Input: part model. Units: mm. Frame: model coordinates. A direction names the side the tool comes from. Round coordinates to 2 decimals unless told otherwise and drop trailing zeros. Order: outer loops, then holes, each group sorted by start corner. A loop starts at its lowest first (then second) coordinate and runs counter-clockwise, first axis right, second up. Notation, with made-up numbers: (12.5, 47) -> (69.5, 47) arc R12 ccw to (69.5, 52) -> close; hole circle Ø3 at (-24, -10.5). An arc over 180 degrees is marked (long way). Answer as CSV lines item,"result". Start each with the question number.
1) Section query A-A, the plane y = 40.5. Output: boundary loops of the cut face in (x, z).
2) Section query B-B, the plane z = 22. Output: boundary loops of the cut face in (x, y).
3) Mould query, pull axis Y, two halves, no side actions, for faces 5 (the face through (26, 3, -10)), 6 (the face through (32.266, 1.479, -13.562)), 7 (the face through (-38.22, 30.225, -8.997)). Classes: +Y half, -Y half, draft (parallel to the pull), parting line (faces both ways), or undercut.
4) Access query for faces 1 (the face through (-40.82, 22.72, -14.99)), 2 (the face through (-31, 3, 13)), 3 (the face through (28.564, 26.856, 9.951)), 4 (the face through (-37.038, 26.856, -6.273)). Directions: +Z, -Z, +X, -X, +Y, -Y. A direction counts if a zero-diameter tool reaches every point of the face in a straight line with its end or side. Return the directions, or none.
5) First-contact query: P1, Ø3, axis at y = 17, z = -10.5, coming from the -X side; P2, Ø4, axis at x = 22, y = 10.5, coming from the -Z side; P3, Ø19, axis at x = 29, z = -21, coming from the +Y side. Flat tips, straight axial feed; report the tip coordinate or a pass-through.
6) Line query: L1, parallel to Y at x = 16, z = -20; L2, parallel to Y at x = -28.5, z = 9; L3, parallel to X at y = 7.5, z = -9. Output: solid intervals per line, ascending.
7) Section query C-C, the plane x = -28. Output: boundary loops of the cut face in (y, z).
```python
from build123d import *

# Parameters (mm, degrees)
SKETCH1_R           = 0.5
BOSS_EXTRUDE1_DEPTH = 3
BOSS_EXTRUDE2_START = 30
SKETCH2_W           = 60
SKETCH2_H           = 40
SKETCH2_R           = 1.689490446
SKETCH2_W_2         = 41
SKETCH2_H_2         = 20.5
BOSS_EXTRUDE2_DEPTH = 3
BOSS_EXTRUDE3_START = -23.72
SKETCH2_2_W         = 60
SKETCH2_2_H         = 40
SKETCH2_2_R         = 1.689490446
SKETCH2_2_W_2       = 41
SKETCH2_2_H_2       = 20.5
BOSS_EXTRUDE3_DEPTH = 3
CUT_EXTRUDE1_DEPTH  = 10


with BuildPart() as part:
    # Sketch1 → Boss-Extrude1 (new body)
    with BuildSketch(Plane(origin=(0, 0, 0), x_dir=(1, 0, 0), z_dir=(0, 1, 0))):
        with BuildLine():
            ThreePointArc((7.77744177, 34.124938088), (-19.979563219, 28.73703279), (-34.697157454, 4.594264319))
            Line((-34.697157454, 4.594264319), (-39.463419759, 15.576857865))
            Line((-39.463419759, 15.576857865), (-42.291947314, 14.577141972))
            Line((-42.291947314, 14.577141972), (-34.916382331, -2.417900937))
            ThreePointArc((-34.916382331, -2.417900937), (-32.106828614, -13.933827771), (-25.614551861, -23.85151427))
            Line((-25.614551861, -23.85151427), (-18.322186149, -40.654846416))
            Line((-18.322186149, -40.654846416), (-15.576857865, -39.463419759))
            Line((-15.576857865, -39.463419759), (-20.34312017, -28.480826213))
            ThreePointArc((-20.34312017, -28.480826213), (7.343177958, -34.221013098), (30.237043308, -17.627286007))
            Line((30.237043308, -17.627286007), (30.950523486, -19.271312771))
            Line((30.950523486, -19.271312771), (33.702537367, -18.076984677))
            Line((33.702537367, -18.076984677), (32.005152982, -14.165810341))
            ThreePointArc((32.005152982, -14.165810341), (32.106828614, 13.933827771), (11.51335986, 33.052118612))
            Line((11.51335986, 33.052118612), (9.815975474, 36.963292947))
            Line((9.815975474, 36.963292947), (7.063961593, 35.768964852))
            Line((7.063961593, 35.768964852), (7.77744177, 34.124938088))
        make_face()
        with Locations(Location((0, -16.15, 0), (0, 0, 270))):
            Circle(SKETCH1_R, mode=Mode.SUBTRACT)
        with BuildLine():
            ThreePointArc((0, -12.65), (0.5, -13.15), (0, -13.65))
            ThreePointArc((0, -13.65), (-0.5, -13.15), (0, -12.65))
        make_face(mode=Mode.SUBTRACT)
        with BuildLine():
            ThreePointArc((0, -9.65), (0.5, -10.15), (0, -10.65))
            ThreePointArc((0, -10.65), (-0.5, -10.15), (0, -9.65))
        make_face(mode=Mode.SUBTRACT)
        with BuildLine():
            ThreePointArc((0, -6.005210608), (0.5, -6.505210608), (0, -7.005210608))
            ThreePointArc((0, -7.005210608), (-0.5, -6.505210608), (0, -6.005210608))
        make_face(mode=Mode.SUBTRACT)
        with Locations(Location((-16.15, 0, 0), (0, 0, 270))):
            Circle(SKETCH1_R, mode=Mode.SUBTRACT)
        with BuildLine():
            ThreePointArc((-13.65, 0), (-13.15, 0.5), (-12.65, 0))
            ThreePointArc((-12.65, 0), (-13.15, -0.5), (-13.65, 0))
        make_face(mode=Mode.SUBTRACT)
        with BuildLine():
            ThreePointArc((-10.65, 0), (-10.15, 0.5), (-9.65, 0))
            ThreePointArc((-9.65, 0), (-10.15, -0.5), (-10.65, 0))
        make_face(mode=Mode.SUBTRACT)
        with BuildLine():
            ThreePointArc((-7.005210608, 0), (-6.505210608, 0.5), (-6.005210608, 0))
            ThreePointArc((-6.005210608, 0), (-6.505210608, -0.5), (-7.005210608, 0))
        make_face(mode=Mode.SUBTRACT)
        with BuildLine():
            ThreePointArc((4.401273885, 0), (3.11217061, -3.11217061), (0, -4.401273885))
            ThreePointArc((0, -4.401273885), (-3.11217061, -3.11217061), (-4.401273885, 0))
            ThreePointArc((-4.401273885, 0), (-3.11217061, 3.11217061), (0, 4.401273885))
            Line((0, 4.401273885), (0, 0))
            Line((0, 0), (4.037455609, 1.752188351))
            ThreePointArc((4.037455609, 1.752188351), (4.309359567, 0.894780386), (4.401273885, 0))
        make_face(mode=Mode.SUBTRACT)
        with BuildLine():
            ThreePointArc((7.005210608, 0), (6.505210608, -0.5), (6.005210608, 0))
            ThreePointArc((6.005210608, 0), (6.505210608, 0.5), (7.005210608, 0))
        make_face(mode=Mode.SUBTRACT)
        with BuildLine():
            ThreePointArc((0, 7.005210608), (0.5, 6.505210608), (0, 6.005210608))
            ThreePointArc((0, 6.005210608), (-0.5, 6.505210608), (0, 7.005210608))
        make_face(mode=Mode.SUBTRACT)
        with BuildLine():
            ThreePointArc((10.65, 0), (10.15, -0.5), (9.65, 0))
            ThreePointArc((9.65, 0), (10.15, 0.5), (10.65, 0))
        make_face(mode=Mode.SUBTRACT)
        with BuildLine():
            ThreePointArc((13.65, 0), (13.15, -0.5), (12.65, 0))
            ThreePointArc((12.65, 0), (13.15, 0.5), (13.65, 0))
        make_face(mode=Mode.SUBTRACT)
        with Locations(Location((16.15, 0, 0), (0, 0, 270))):
            Circle(SKETCH1_R, mode=Mode.SUBTRACT)
        with BuildLine():
            ThreePointArc((0, 10.65), (0.5, 10.15), (0, 9.65))
            ThreePointArc((0, 9.65), (-0.5, 10.15), (0, 10.65))
        make_face(mode=Mode.SUBTRACT)
        with BuildLine():
            ThreePointArc((0, 13.65), (0.5, 13.15), (0, 12.65))
            ThreePointArc((0, 12.65), (-0.5, 13.15), (0, 13.65))
        make_face(mode=Mode.SUBTRACT)
        with Locations(Location((0, 16.15, 0), (0, 0, 270))):
            Circle(SKETCH1_R, mode=Mode.SUBTRACT)
    extrude(amount=BOSS_EXTRUDE1_DEPTH)

    # Sketch2 → Boss-Extrude2 (add)
    with BuildSketch(Plane(origin=(0, 0, 0), x_dir=(0.3981093648941227, 0, 0.9173379603960573), z_dir=(-0.9173379603960573, 0, 0.3981093648941227)).offset(BOSS_EXTRUDE2_START)):
        with Locations((0, 23)):
            Rectangle(SKETCH2_W, SKETCH2_H)
        with Locations(Location((-23.689490446, 31.9, 0), (0, 0, 180))):
            Circle(SKETCH2_R, mode=Mode.SUBTRACT)
        with Locations(Location((-23.689490446, 22.1, 0), (0, 0, 180))):
            Circle(SKETCH2_R, mode=Mode.SUBTRACT)
        with Locations(Location((23.689490446, 22.1, 0), (0, 0, 180))):
            Circle(SKETCH2_R, mode=Mode.SUBTRACT)
        with Locations(Location((23.689490446, 31.9, 0), (0, 0, 180))):
            Circle(SKETCH2_R, mode=Mode.SUBTRACT)
        with Locations((0, 27)):
            Rectangle(SKETCH2_W_2, SKETCH2_H_2, mode=Mode.SUBTRACT)
    extrude(amount=BOSS_EXTRUDE2_DEPTH)

    # Sketch2<2> → Boss-Extrude3 (add)
    with BuildSketch(Plane(origin=(0, 0, 0), x_dir=(0.3981093648941227, 0, 0.9173379603960573), z_dir=(-0.9173379603960573, 0, 0.3981093648941227)).offset(BOSS_EXTRUDE3_START)):
        with Locations((0, 23)):
            Rectangle(SKETCH2_2_W, SKETCH2_2_H)
        with Locations(Location((-23.689490446, 31.9, 0), (0, 0, 180))):
            Circle(SKETCH2_2_R, mode=Mode.SUBTRACT)
        with Locations(Location((-23.689490446, 22.1, 0), (0, 0, 180))):
            Circle(SKETCH2_2_R, mode=Mode.SUBTRACT)
        with Locations(Location((23.689490446, 22.1, 0), (0, 0, 180))):
            Circle(SKETCH2_2_R, mode=Mode.SUBTRACT)
        with Locations(Location((23.689490446, 31.9, 0), (0, 0, 180))):
            Circle(SKETCH2_2_R, mode=Mode.SUBTRACT)
        with Locations((0, 27)):
            Rectangle(SKETCH2_2_W_2, SKETCH2_2_H_2, mode=Mode.SUBTRACT)
    extrude(amount=BOSS_EXTRUDE3_DEPTH)

    # Sketch1<3> → Cut-Extrude1 (cut)
    with BuildSketch(Plane(origin=(0, 0, 0), x_dir=(1, 0, 0), z_dir=(0, 1, 0))):
        with BuildLine():
            Line((0, 4.401273885), (0, 0))
            Line((0, 0), (4.037455609, 1.752188351))
            ThreePointArc((4.037455609, 1.752188351), (2.414472094, 3.679882651), (0, 4.401273885))
        make_face()
    extrude(amount=CUT_EXTRUDE1_DEPTH, mode=Mode.SUBTRACT)


solid = part.part
```
Findings:
1,outline,"(-42.22, -14.38) -> (-39.46, -15.58) -> (-15.58, 39.46) -> (-18.33, 40.66) -> close; (7.06, -35.77) -> (9.82, -36.96) -> (33.7, 18.08) -> (30.95, 19.27) -> close"
2,outline,"(-27.22, 0) -> (27.22, 0) -> (27.22, 3) -> (-23.16, 3) -> (-23.16, 16.75) -> (-26.43, 16.75) -> (-26.43, 3) -> (-27.22, 3) -> close; (-26.43, 37.25) -> (-23.16, 37.25) -> (-23.16, 43) -> (-26.43, 43) -> close"
3,face 5,"+Y half"
3,face 6,"draft"
3,face 7,"undercut"
4,face 1,"-Z, -X, +Y"
4,face 2,"+Z, -X, +Y"
4,face 3,"-Z, -X"
4,face 4,"+Z, +X"
5,P1,"stops at x = -41.18"
5,P2,"stops at z = -13.5"
5,P3,"stops at y = 3"
6,L1,"y = 0 to 16.75, 37.25 to 43"
6,L2,"y = 0 to 3"
6,L3,"x = -39.88 to -36.61, 18.68 to 21.95"
7,outline,"(0, -21) -> (3, -21) -> (3, 10.84) -> (16.75, 10.84) -> (16.75, 18.37) -> (3, 18.37) -> (3, 21) -> (0, 21) -> close; (37.25, 10.84) -> (43, 10.84) -> (43, 18.37) -> (37.25, 18.37) -> close"
